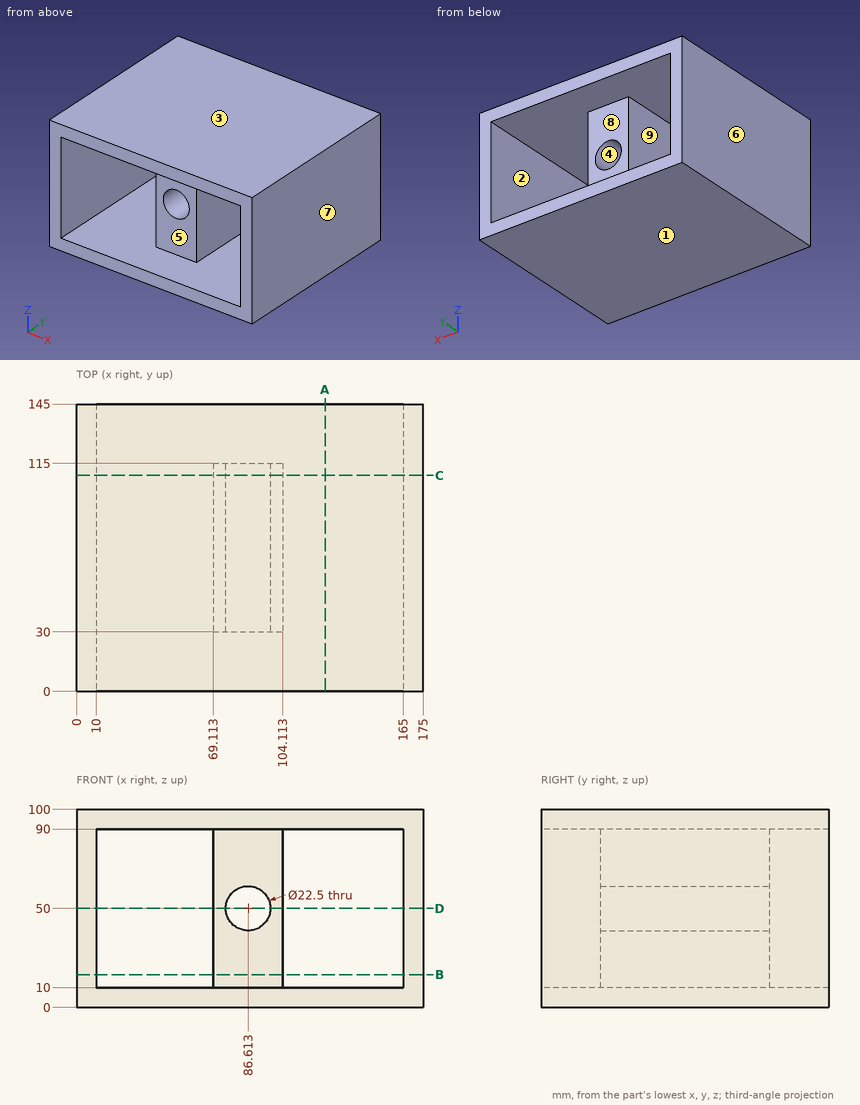
Part print with two shaded views. Sizes in mm from the minimum x, y, z corner. A direction names the side the tool comes from. Give positions to 0.01 mm unless a question says otherwise; leave off trailing zeros. Write each loop counter-clockwise with the first axis right and the second up, starting at its lowest first coordinate (ties: lowest second). Pieces come first, ordered by that corner, then holes.
1) Cut at D-D on z = 50. Write the cut outline in (x, y).
Resolved:
outline: (0, 0) - (10, 0) - (10, 145) - (0, 145) - close; (69.11, 30) - (75.36, 30) - (75.36, 115) - (69.11, 115) - close; (97.86, 30) - (104.11, 30) - (104.11, 115) - (97.86, 115) - close; (165, 0) - (175, 0) - (175, 145) - (165, 145) - close
2) Which spindle directions (+Z, -Z, +X, -X, +Y, -Y) get a long thin tool onto all of the face, cutting with end or side? Do the marked faces 5, 6, 7, 8 and 9. Say none if no direction does.
Resolved:
face 5: -Y
face 6: +Z, -Z, -X, +Y, -Y
face 7: +Z, -Z, +X, +Y, -Y
face 8: +Y
face 9: +Y, -Y
3) Probe L1, parallel to X at y = 69, z = 11.5; L2, parallel to X at y = 87, z = 50; L3, parallel to Z at x = 111, y = 32. List the from-to ranges inside material, lowest first.
Resolved:
L1: x = 0 to 10, 69.11 to 104.11, 165 to 175
L2: x = 0 to 10, 69.11 to 75.36, 97.86 to 104.11, 165 to 175
L3: z = 0 to 10, 90 to 100
4) Cut at A-A on x = 125.5. Write the cut outline in (y, z), then the cut area to 3 significant figures.
Resolved:
outline: (0, 0) - (145, 0) - (145, 10) - (0, 10) - close; (0, 90) - (145, 90) - (145, 100) - (0, 100) - close
area: 2,900 mm2
5) Cut at C-C on y = 109. Write the cut outline in (x, z), then the cut area to 3 significant figures.
Resolved:
outline: (0, 0) - (175, 0) - (175, 100) - (0, 100) - close; hole (10, 10) - (69.11, 10) - (69.11, 90) - (10, 90) - close; hole circle Ø22.5 at (86.61, 50); hole (104.11, 10) - (165, 10) - (165, 90) - (104.11, 90) - close
area: 7,500 mm2
6) Cut at B-B on z = 16.5. Write the cut outline in (x, y).
Resolved:
outline: (0, 0) - (10, 0) - (10, 145) - (0, 145) - close; (69.11, 30) - (104.11, 30) - (104.11, 115) - (69.11, 115) - close; (165, 0) - (175, 0) - (175, 145) - (165, 145) - close
7) Two-plate mould, pull along Z, no slides. Class the marked faces 1, 2, 3 and 4: released by +Z, released by -Z, zero draft, split by the parting line, or undercut.
Resolved:
face 1: released by -Z
face 2: undercut
face 3: released by +Z
face 4: undercut
